Input: dimensioned drawing with shaded views. Units: mm. Origin: part minimum x, y, z. A direction names the side the tool comes from. Round coordinates to 2 decimals unless told otherwise and drop trailing zeros. Loops run counter-clockwise (first coordinate to the right, second up) from the corner with the lowest first, then second, coordinate; pieces in that order, holes last. Notation, with made-up numbers: (73, 41) -> (87, 41) arc R8 cw to (87, 52) -> close; hole circle Ø8 at (67, 44). An arc over 180 degrees is marked (long way). Answer as a JSON object with one key per item and string values.
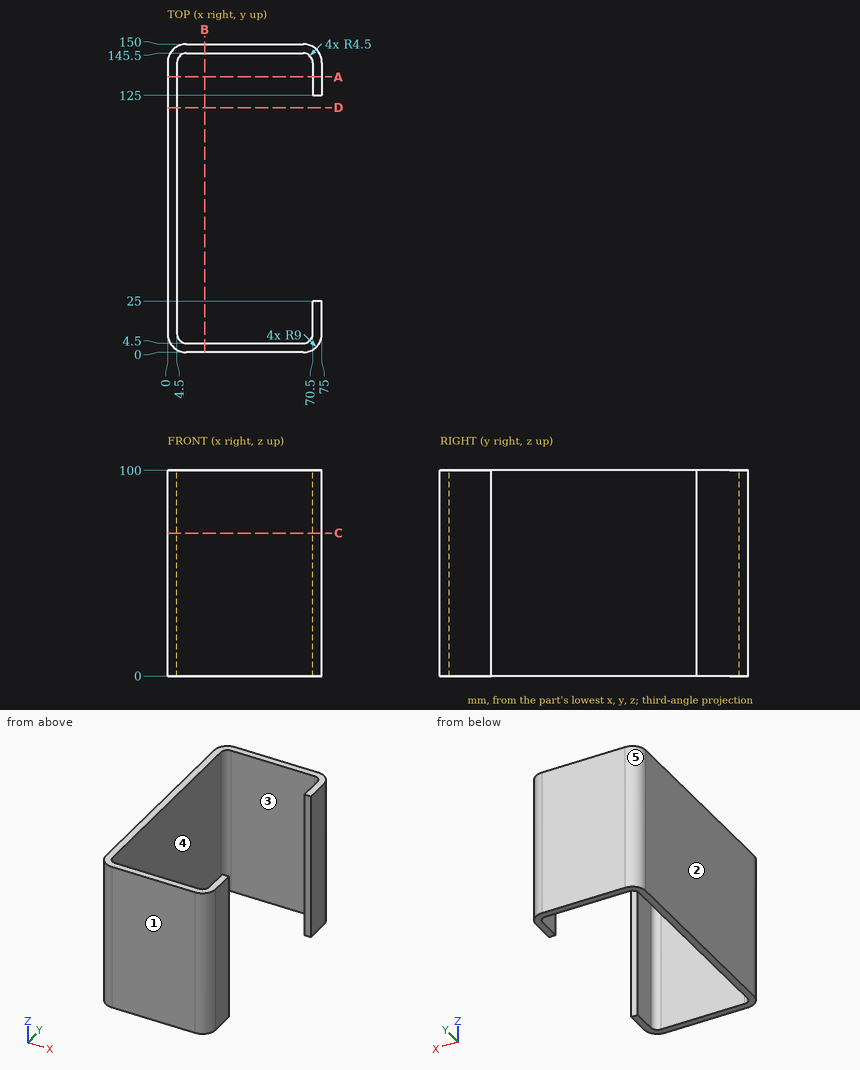
1) Section C-C, the plane z = 69.5. Output: boundary loops of the cut face in (x, y).
Output:
{"outline": "(0, 9) arc R9 ccw to (9, 0) -> (66, 0) arc R9 ccw to (75, 9) -> (75, 25) -> (70.5, 25) -> (70.5, 9) arc R4.5 cw to (66, 4.5) -> (9, 4.5) arc R4.5 cw to (4.5, 9) -> (4.5, 141) arc R4.5 cw to (9, 145.5) -> (66, 145.5) arc R4.5 cw to (70.5, 141) -> (70.5, 125) -> (75, 125) -> (75, 141) arc R9 ccw to (66, 150) -> (9, 150) arc R9 ccw to (0, 141) -> close"}
2) Ray query, probe 1 along X at (y, z) = (132, 33.5); probe 2 along Y at (x, z) = (19.5, 68.5); probe 3 along X at (y, z) = (108.5, 15). Return the intervals inside material, ascending.
Output:
{"probe 1": "x = 0 to 4.5, 70.5 to 75", "probe 2": "y = 0 to 4.5, 145.5 to 150", "probe 3": "x = 0 to 4.5"}
3) Draft query along Y for the marked faces 1, 2 and 3. Return one class per face: +Y half, -Y half, draft (parallel to the pull), parting line (faces both ways), or undercut.
Output:
{"face 1": "-Y half", "face 2": "draft", "face 3": "undercut"}
4) Section A-A, the plane y = 134. Output: boundary loops of the cut face in (x, z), plus the area to 3 significant figures.
Output:
{"outline": "(0, 0) -> (4.5, 0) -> (4.5, 100) -> (0, 100) -> close; (70.5, 0) -> (75, 0) -> (75, 100) -> (70.5, 100) -> close", "area": "900 mm^2"}
5) Section B-B, the plane x = 18. Output: boundary loops of the cut face in (y, z), plus the area to 3 significant figures.
Output:
{"outline": "(0, 0) -> (4.5, 0) -> (4.5, 100) -> (0, 100) -> close; (145.5, 0) -> (150, 0) -> (150, 100) -> (145.5, 100) -> close", "area": "900 mm^2"}
6) Reachability of the marked faces 4 and 5 from +Z, -Z, +X, -X, +Y, -Y: full face, straight path, thin tool, end or side. Return the list, or none.
Output:
{"face 4": "+Z, -Z", "face 5": "+Z, -Z, -X, +Y"}
7) Contact query for flat-ended pins moving along their axis: P1, Ø2, axis at x = 73, z = 32, coming from the -Y side; P2, Ø3.5, axis at x = 72.5, z = 54, coming from the +Y side; P3, Ø12, axis at y = 101.5, z = 89, coming from the +X side. Output: stop coordinate, or through.
Output:
{"P1": "stops at y = 2.29", "P2": "stops at y = 148.64", "P3": "stops at x = 4.5"}
8) Section D-D, the plane y = 119. Output: boundary loops of the cut face in (x, z).
Output:
{"outline": "(0, 0) -> (4.5, 0) -> (4.5, 100) -> (0, 100) -> close"}
